Check sheet for the modelled part. Datum: model origin and axes. Units: mm. Face numbers are marked on the shaded views. Give positions to 0.01 mm unless a question says otherwise; leave off trailing zeros. Order: outer loops, then holes, each group sorted by start corner. A loop starts at its lowest first (then second) coordinate and runs counter-clockwise, first axis right, second up. Notation, with made-up numbers: (41, 29.25) - (73, 29.25) arc R12 cw to (73, 44.25) - close; hole circle Ø4 at (45.25, 37). An arc over 180 degrees is marked (long way). Answer in a Markdown table with one row per item.
from build123d import *

# Parameters (mm, degrees)
F0_R     = 60
F2_R     = 11
F4_DEPTH = 35
F5_T     = -2


with BuildPart() as f3:
    # F0 (on Top) → F3 section 0
    with BuildSketch(Plane.XY):
        Circle(F0_R)
    # F2 (on offset) → F3 section 1
    with BuildSketch(Plane.XY.offset(-70)):
        Circle(F2_R)
    loft()

    # F4 (add): a face of the model
    f4_faces = [f3.faces().sort_by_distance(p)[0] for p in [
        (0, 0, -70),
    ]]
    extrude(f4_faces, amount=F4_DEPTH)

    # F5
    f5_openings = [f3.faces().sort_by_distance(p)[0] for p in [
        (0, 0, 0),
        (0, 0, -105),
    ]]
    offset(amount=F5_T, openings=f5_openings, kind=Kind.INTERSECTION)


solid = f3.part
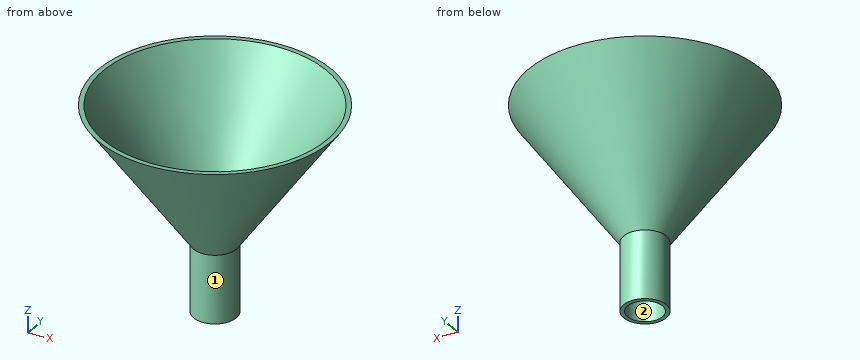
(1) Cross-section at B-B, the plane z = -95.5. Record the cut outline in (x, y), then the cut area to 3 significant figures.
Geometry says:
| item | result |
|---|---|
| outline | circle Ø22 at (0, 0); hole circle Ø18 at (0, 0) |
| area | 126 mm² |
(2) Cross-section at C-C, the plane z = -46. Record the cut outline in (x, y), then the cut area to 3 significant figures.
Geometry says:
| item | result |
|---|---|
| outline | circle Ø55.6 at (0, 0); hole circle Ø50.72 at (0, 0) |
| area | 408 mm² |
(3) Thickness scan on L1, parallel to Y at x = 0, z = -86; L2, parallel to Y at x = 18, z = -6.5; L3, parallel to Z at x = -54, y = -11.5. Record the ranges inside material, lowest first.
Geometry says:
| item | result |
|---|---|
| L1 | -11 to -9, 9 to 11 |
| L2 | -52.45 to -49.86, 49.86 to 52.45 |
| L3 | -6.84 to -3.35 |
(4) Mould release check, pull along X, two halves, no side actions. Record for the marked faces 1 and 2: pulls with the +X half, pulls with the -X half, needs draft (parallel to the pull), parting line crosses it, or undercut.
Geometry says:
| item | result |
|---|---|
| face 1 | parting line crosses it |
| face 2 | undercut |
(5) Cross-section at A-A, the plane x = 0. Record the cut outline in (y, z), then the cut area to 3 significant figures.
Geometry says:
| item | result |
|---|---|
| outline | (-60, 0) - (-11, -70) - (-11, -105) - (-9, -105) - (-9, -69.37) - (-57.56, 0) - close; (9, -105) - (11, -105) - (11, -70) - (60, 0) - (57.56, 0) - (9, -69.37) - close |
| area | 482 mm² |
(6) Gauge pin test, flat ends, axial feed: P1, Ø3, axis at y = -2, z = -28, coming from the -X side; P2, Ø2, axis at x = 47.5, y = 13.5, coming from the +Z side; P3, Ø3, axis at x = 41, y = -18.5, coming from the +Z side; P4, Ø23.5, axis at x = 0, y = 0, coming from the -Z side. Record the tip position at first contact, or that the pin passes through.
Geometry says:
| item | result |
|---|---|
| P1 | x = -41.4 |
| P2 | z = -10.25 |
| P3 | z = -15.83 |
| P4 | z = -105 |
